from build123d import *

# Parameters (mm, degrees)
F0_W     = 480
F0_H     = 1110
F1_DEPTH = 350
F2_T     = -10


# Not quite as in the source:
# - the program builds the solid bodies; features that only make, move or delete a surface that nothing else refers to are left out


with BuildPart() as f1:
    # F0 (on Top) → F1 (new body, symmetric)
    with BuildSketch(Plane.XY):
        Rectangle(F0_W, F0_H)
    extrude(amount=F1_DEPTH, both=True)

    # F2 (hollow: no face is removed)
    offset(amount=F2_T, mode=Mode.SUBTRACT)


solid = f1.part
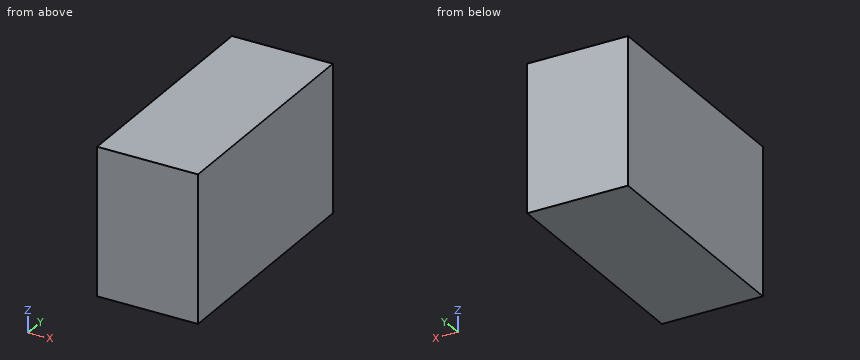
The listing builds one solid part. Answer for the finished solid, in the listing's coordinates (mm). Give positions to 0.01 mm unless a question says otherwise; leave off trailing zeros. Loops run counter-clockwise (first coordinate to the right, second up) from the corner with the lowest first, then second, coordinate; pieces in that order, holes last.
Item 1: A cutting plane is placed at B-B (z = 253). Give the vertices of the cut face in (x, y).
Derived:
outline: (-240, -555) - (240, -555) - (240, 555) - (-240, 555) - close; hole (-230, -545) - (230, -545) - (230, 545) - (-230, 545) - close
Item 2: A cutting plane is placed at A-A (x = 182.5). Give the vertices of the cut face in (y, z).
Derived:
outline: (-555, -350) - (555, -350) - (555, 350) - (-555, 350) - close; hole (-545, -340) - (545, -340) - (545, 340) - (-545, 340) - close
Item 3: Find the intervals of material crossed by line 1 along Y through (x, z) = (54, -67); line 2 along X through (y, z) = (-243.5, -185); line 3 along Z through (x, y) = (-114, 61), in increasing order.
Derived:
line 1: y = -555 to -545, 545 to 555
line 2: x = -240 to -230, 230 to 240
line 3: z = -350 to -340, 340 to 350
